Work out the finished part from the listing and answer in its coordinate system (mm). A direction names the side the tool comes from. Coordinates: 2 decimals unless noted, no trailing zeros. Order: outer loops, then holes, each group sorted by start corner. A loop starts at its lowest first (then second) coordinate and runs counter-clockwise, first axis right, second up. Notation, with made-up numbers: (-4.5, 8.5) -> (32.5, 8.5) arc R11 cw to (32.5, 26.5) -> close; hole circle Ø9 at (72, 67.5). An arc over 180 degrees is marked (long way). Write item = value, one per line. Start each with the question number.
Q1. Straight lines are drawn through the part: L1, parallel to Z at x = 100.5, y = 1706; L2, parallel to Y at x = -21.5, z = -6.5; L3, parallel to Z at x = 68.5, y = 1931. For each, find the intervals that lie inside material, in ascending order. Write a range as from..to.
Q2. The part is cut by section B-B, the plane z = -55. Determine the outline of the cut face in (x, y).
Q3. Flat-ended cylindrical pins translate along their axes: pin 1 (3 mm diameter, centred on x = 82, z = 10, fed in from -Y); pin 2 (10 mm diameter, centred on x = -4.5, y = 720.5, fed in from -Z); pin 3 (12 mm diameter, centred on x = -69, z = -75, fed in from -Y). Find the tip coordinate at first contact, or state that the pin passes through.
Q4. The part is cut by section C-C, the plane z = 73. Determine the outline of the cut face in (x, y), plus the area to 3 significant figures.
Q5. The part is cut by section D-D, the plane y = 1273.5. Determine the outline of the cut face in (x, z).
Q6. For a pull along Y with two mould halves and no side action, classify faces 1 (the cylindrical face through (-2.529, 2018.702, 49.3)), 2 (the cylindrical face through (-9.764, 74.362, -101.746)), 3 (the flat face through (2, 967, 100)), 4 (the flat face through (2, 967, 0)) as +Y half, -Y half, draft (parallel to the pull), parting line (faces both ways), or undercut.
Q7. The part is cut by section A-A, the plane x = -28.5. Determine the outline of the cut face in (y, z).
Q8. Which of the six approach directions +Z, -Z, +X, -X, +Y, -Y give full straight-line access (tool end or side, diameter ignored) to faces 5 (the flat face through (-1, 1, -206.381)), 6 (the flat face through (-1, 1905, -83.1)), 7 (the cylindrical face through (95.38, 1933.77, -40.97))?
```python
from build123d import *

# Parameters (mm, degrees)
BOSS_EXTRUDE1_DEPTH = 100
SKETCH1_4_R         = 100
BOSS_EXTRUDE3_DEPTH = 83.10006502
SKETCH1_5_R         = 75
BOSS_EXTRUDE4_DEPTH = 206.380604418


with BuildPart() as part:
    # Sketch1 → Boss-Extrude1 (new body)
    with BuildSketch(Plane.XY):
        with BuildLine():
            Line((-115, 0), (-115, 1903.73))
            ThreePointArc((-115, 1903.73), (0, 2018.73), (115, 1903.73))
            Line((115, 1903.73), (115, 0))
            ThreePointArc((115, 0), (0, -115), (-115, 0))
        make_face()
    extrude(amount=BOSS_EXTRUDE1_DEPTH)

    # Sketch1<4> → Boss-Extrude3 (add)
    with BuildSketch(Plane.XY):
        with Locations((0, 1903.73)):
            Circle(SKETCH1_4_R)
    extrude(amount=-BOSS_EXTRUDE3_DEPTH)

    # Sketch1<5> → Boss-Extrude4 (add)
    with BuildSketch(Plane.XY):
        Circle(SKETCH1_5_R)
    extrude(amount=-BOSS_EXTRUDE4_DEPTH)


solid = part.part
```
Model answer:
q1.L1 = 0..100
q1.L2 = -71.85..71.85, 1806.07..2001.39
q1.L3 = -83.1..100
q2.outline = circle Ø200 at (0, 1903.73); circle Ø150 at (0, 0)
q3.pin_1 = -82.13
q3.pin_2 = 0
q3.pin_3 = -40.69
q4.outline = (-115, 0) arc R115 ccw to (115, 0) -> (115, 1903.73) arc R115 ccw to (-115, 1903.73) -> close
q4.area = 479,000 mm2
q5.outline = (-115, 0) -> (115, 0) -> (115, 100) -> (-115, 100) -> close
q6.face_1 = +Y half
q6.face_2 = undercut
q6.face_3 = draft
q6.face_4 = undercut
q7.outline = (-111.41, 0) -> (-69.37, 0) -> (-69.37, -206.38) -> (69.37, -206.38) -> (69.37, 0) -> (1807.88, 0) -> (1807.88, -83.1) -> (1999.58, -83.1) -> (1999.58, 0) -> (2015.14, 0) -> (2015.14, 100) -> (-111.41, 100) -> close
q8.face_5 = -Z, +X, -X, +Y, -Y
q8.face_6 = -Z, +X, -X, +Y
q8.face_7 = -Z
